Autodesk Inventor part; units mm, degrees
ref_plane "YZ Plane" through (0, 0, 0) normal (1, 0, 0) x (0, 1, 0)
ref_plane "XZ Plane" through (0, 0, 0) normal (0, 1, 0) x (-1, 0, 0)
ref_plane "XY Plane" through (0, 0, 0) normal (0, 0, 1) x (1, 0, 0)
sketch "Esquisse1" plane through (0, 0, 0) normal (0, 1, 0) x (-1, 0, 0)
  line L0 (-225, -262.5) -> (225, -262.5)
  line L1 (225, -262.5) -> (225, 262.5)
  line L2 (225, 262.5) -> (-225, 262.5)
  line L3 (-225, 262.5) -> (-225, -262.5)
  line L4 (-225, -262.5) -> (225, 262.5) construction
  line L5 (225, -262.5) -> (-225, 262.5) construction
  point P0 (0, 0)
  dimension "d0" = 525
  dimension "d1" = 450
extrude "Extrusion1" add sketch "Esquisse1" along normal blind 290
sketch "Esquisse2" plane through (0, 290, 0) normal (0, 1, 0) x (1, 0, 0)
  line L0 (-343, 683) -> (-343, -411)
  line L1 (-343, -411) -> (-308, -411)
  line L2 (373, -411) -> (373, 683)
  line L3 (-308, -411) -> (-308, -271)
  line L4 (-308, -271) -> (338, -271)
  line L5 (338, -271) -> (338, -411)
  line L6 (-308, 683) -> (-308, 302)
  line L7 (-308, 302) -> (338, 302)
  line L8 (338, 302) -> (338, 683)
  line L9 (373, 683) -> (338, 683)
  line L10 (-308, 683) -> (-343, 683)
  line L11 (338, -411) -> (373, -411)
  line L12 (-225, 262.5) -> (-225, -262.5) construction
  line L13 (225, -262.5) -> (225, 262.5) construction
  line L14 (225, 262.5) -> (-225, 262.5) construction
  line L15 (-225, -262.5) -> (225, -262.5) construction
  point P0 (0, 0)
  dimension "d4" = 646
  dimension "d5" = 573
  dimension "d6" = 140
  dimension "d7" = 381
  dimension "d8" = 35
  dimension "d9" = 35
  dimension "d10" = 118
  dimension "d11" = 148
  dimension "d12" = 1094
  dimension "d13" = 39.5
  dimension "d14" = 8.5
  dimension "d15" = 525
extrude "Extrusion2" add sketch "Esquisse2" along normal blind 40
sketch "Esquisse3" plane through (338, 290, 411) normal (0, 0, 1) x (1, 0, 0)
  line L0 (-646, 0) -> (0, 0)
  line L1 (-646, 0) -> (-649, 0)
  line L2 (-649, 0) -> (-649, -19)
  line L3 (-649, -19) -> (-646, -19)
  line L4 (-646, -19) -> (-646, 0)
  line L5 (0, 0) -> (35, 0)
  line L6 (0, 0) -> (3, 0)
  line L7 (3, 0) -> (3, -19)
  line L8 (3, -19) -> (0, -19)
  line L9 (0, -19) -> (0, 0)
  line L10 (0, 40) -> (35, 40)
  point P0 (-338, -290)
  point P1 (3, 0)
  dimension "d18" = 59
  dimension "d19" = 3
extrude "Extrusion3" add sketch "Esquisse3" against normal blind 1093
sketch "Esquisse4" plane through (-225, 0, -262.5) normal (-1, 0, 0) x (0, 0, 1)
  circle A0 centre (255, 80) radius 40
  line L0 (0, 0) -> (0, 290)
  line L1 (0, 0) -> (525, 0)
  line L2 (525, 0) -> (525, 290)
  point P0 (262.5, 0)
  dimension "d23" = 80
  dimension "d24" = 255
  dimension "d25" = 80
  dimension "d26" = 270
extrude "Extrusion4" add sketch "Esquisse4" along normal blind 110
sketch "Esquisse5" plane through (225, 0, -262.5) normal (0, 0, -1) x (-1, 0, 0)
  line L0 (0, 0) -> (0, 290)
  line L1 (0, 290) -> (110, 290)
  line L2 (110, 290) -> (110, 200)
  line L3 (110, 200) -> (0, 200)
  line L4 (0, 200) -> (0, 290)
  point P0 (225, 0)
  point P1 (0, 200)
  dimension "d29" = 90
  dimension "d30" = 110
extrude "Extrusion5" add sketch "Esquisse5" along normal blind 30
sketch "Esquisse6" plane through (225, 0, 262.5) normal (1, 0, 0) x (0, 0, -1)
  circle A0 centre (160, 60) radius 60
  line L0 (0, 0) -> (0, 290)
  line L1 (0, 0) -> (525, 0)
  point P0 (262.5, 0)
  dimension "d33" = 120
  dimension "d34" = 160
  dimension "d35" = 60
extrude "Extrusion6" add sketch "Esquisse6" along normal blind 100
sketch "Esquisse8" plane through (225, 0, 262.5) normal (1, 0, 0) x (0, 0, -1)
  circle A0 centre (380, 271) radius 25
  line L0 (525, 0) -> (525, 200)
  line L1 (-148.5, 271) -> (944.5, 271)
  point P0 (262.5, 0)
  point P1 (945.5, 271)
  dimension "d38" = 50
  dimension "d39" = 145
extrude "Extrusion7" add sketch "Esquisse8" along normal blind 160
sketch "Esquisse9" plane through (-225, 0, -262.5) normal (-1, 0, 0) x (0, 0, 1)
  arc A0 (128.7519, 290) -> (161.2481, 290) centre (145, 271) ccw
  circle A1 centre (145, 271) radius 22.5
  point P0 (262.5, 0)
  dimension "d42" = 45
extrude "Extrusion8" add sketch "Esquisse9" along normal blind 110
ref_plane "Plan de construction1" through (15, 290, -683) normal (1, 0, 0) x (0, 0, -1)
ref_plane "Plan de construction2" through (338, 290, -15.5) normal (0, 0, -1) x (-1, 0, 0)
ref_plane "Plan de construction3" through (413, 290, -683) normal (1, 0, 0) x (0, 0, -1)
sketch "Esquisse10" plane through (413, 290, -683) normal (1, 0, 0) x (0, 0, -1)
  line L0 (-620.5, 0) -> (-710.5, 0)
  line L1 (-710.5, 0) -> (-710.5, 95)
  line L2 (-710.5, 95) -> (-620.5, 95)
  line L3 (-620.5, 95) -> (-620.5, 0)
  line L4 (-549.2519, 0) -> (0, 0)
  line L5 (-390.5, 0) -> (-390.5, -90)
  line L6 (-420.5, -290) -> (-420.5, -90)
  point P0 (-683, -290)
  dimension "d46" = 90
  dimension "d47" = 95
  dimension "d50" = 200
extrude "Extrusion9" add sketch "Esquisse10" against normal blind 796
sketch "Esquisse11" plane through (-343, 290, -683) normal (-1, 0, 0) x (0, 0, 1)
  line L0 (577.552, 0) -> (945.5, 0)
  line L1 (785, 40) -> (809, 40)
  line L2 (809, 40) -> (809, 29)
  line L3 (809, 29) -> (785, 29)
  line L4 (785, 29) -> (785, 40)
  line L5 (945.5, -290) -> (945.5, 0)
  line L6 (710.5, 40) -> (1094, 40)
  line L7 (620.5, 40) -> (0, 40)
  line L8 (512, 40) -> (536, 40)
  line L9 (536, 40) -> (536, 29)
  line L10 (536, 29) -> (512, 29)
  line L11 (512, 29) -> (512, 40)
  line L12 (420.5, -290) -> (420.5, 0)
  line L13 (381, 0) -> (381, 40)
  point P0 (683, -290)
  point P1 (954, 40)
  dimension "d52" = 24
  dimension "d53" = 11
  dimension "d57" = 131
  dimension "d58" = 145
extrude "Extrusion10" cut sketch "Esquisse11" against normal blind 776
properties part number "SAW_DM"
Verification items for the finished model (mm, model axes). A direction names the side the tool comes from. Coordinates: 2 decimals unless noted, no trailing zeros. Order: outer loops, then holes, each group sorted by start corner. A loop starts at its lowest first (then second) coordinate and runs counter-clockwise, first axis right, second up. Notation, with made-up numbers: M -9.5,36 L 11.5,36 A35 ccw 11.5,72 Z; hole C 61.25,52.25 d8. An arc over 180 degrees is marked long. Return JSON: item names as keys, results as strings.
1) Gauge pin test, flat ends, axial feed: pin 1 (10 mm diameter, centred on y = 41.5, z = -62, fed in from +X); pin 2 (1 mm diameter, centred on y = 320, z = 168.5, fed in from -X); pin 3 (1.5 mm diameter, centred on y = 291.5, z = -468, fed in from +X). Record the tip position at first contact, or that the pin passes through.
Answer list:
{"pin 1": "x = 225", "pin 2": "x = -343", "pin 3": "x = 373"}
2) Cross-section at B-B, the plane z = -476. Record the boundary of the cut face in (x, y).
Answer list:
{"outline": "M -343,290 L -311,290 L -311,271 L -308,271 L -308,330 L -343,330 Z; M 338,271 L 341,271 L 341,290 L 373,290 L 373,330 L 338,330 Z"}
3) Cross-section at C-C, the plane z = -7.5. Record the boundary of the cut face in (x, y).
Answer list:
{"outline": "M -383,290 L -311,290 L -311,271 L -308,271 L -308,290 L -225,290 L -225,120 L -335,120 L -335,40 L -225,40 L -225,0 L 225,0 L 225,290 L 338,290 L 338,271 L 341,271 L 341,290 L 413,290 L 413,385 L -383,385 Z"}
4) Release check for a two-part mould opening along X. For faces 1 (the flat face through (10, 330, 203)), 2 (the flat face through (10, 290, -274)), 3 (the flat face through (-335, 270, -118)) record: +X half, -X half, draft (parallel to the pull), parting line (faces both ways), or undercut.
Answer list:
{"face 1": "draft", "face 2": "undercut", "face 3": "-X half"}
5) Cross-section at D-D, the plane y = 138.5. Record the boundary of the cut face in (x, z), and give its area (3 significant figures).
Answer list:
{"outline": "M -225,-262.5 L 225,-262.5 L 225,262.5 L -225,262.5 Z", "area": "236,000 mm2"}
6) Access from +Z, -Z, +X, -X, +Y, -Y to the whole of each face (thin tool, end or side, straight path). Record for faces 4 (the flat face through (373, 310, 222)), 5 (the flat face through (115, 246, -277)), 6 (the flat face through (10, 310, 271)).
Answer list:
{"face 4": "+Z, +X, +Y, -Y", "face 5": "-Z, -Y", "face 6": "+Z, +Y, -Y"}
7) Thickness scan on L1, parallel to Z at x = -256, y = 329; L2, parallel to X at y = 317.5, z = -505; L3, parallel to Z at x = -121.5, y = 211.5. Record the ranges inside material, lowest first. Write a range as [from, to].
Answer list:
{"L1": "[-302, -171], [-147, 102], [126, 271]", "L2": "[-343, -308], [338, 373]", "L3": "[-262.5, 262.5]"}
8) Cross-section at A-A, the plane x = 46. Record the boundary of the cut face in (y, z), and give its area (3 significant figures).
Answer list:
{"outline": "M 0,-262.5 L 290,-262.5 L 290,-302 L 330,-302 L 330,-171 L 319,-171 L 319,-147 L 330,-147 L 330,-62.5 L 385,-62.5 L 385,27.5 L 330,27.5 L 330,102 L 319,102 L 319,126 L 330,126 L 330,271 L 290,271 L 290,262.5 L 0,262.5 Z", "area": "180,000 mm2"}
